from build123d import *

# Parameters (mm, degrees)
SKETCH1_R           = 17
BOSS_EXTRUDE1_DEPTH = 10


with BuildPart() as part:
    # Sketch1 → Boss-Extrude1 (new body)
    with BuildSketch(Plane(origin=(0, 0, 0), x_dir=(1, 0, 0), z_dir=(0, 1, 0))):
        with BuildLine():
            Line((-24.933996638, 20), (12.2, 20))
            ThreePointArc((12.2, 20), (-11.288251879, 45.878391012), (-39.314701644, 25))
            Line((-39.314701644, 25), (-164.9, 25))
            ThreePointArc((-164.9, 25), (-189.9, 0), (-164.9, -25))
            Line((-164.9, -25), (-39.314701644, -25))
            ThreePointArc((-39.314701644, -25), (-11.288251879, -45.878391012), (12.2, -20))
            Line((12.2, -20), (-24.933996638, -20))
            ThreePointArc((-24.933996638, -20), (-31.954004645, 0), (-24.933996638, 20))
        make_face()
        with Locations(Location((-164.9, 0, 0), (0, 0, 270))):
            Circle(SKETCH1_R, mode=Mode.SUBTRACT)
    extrude(amount=BOSS_EXTRUDE1_DEPTH)


solid = part.part
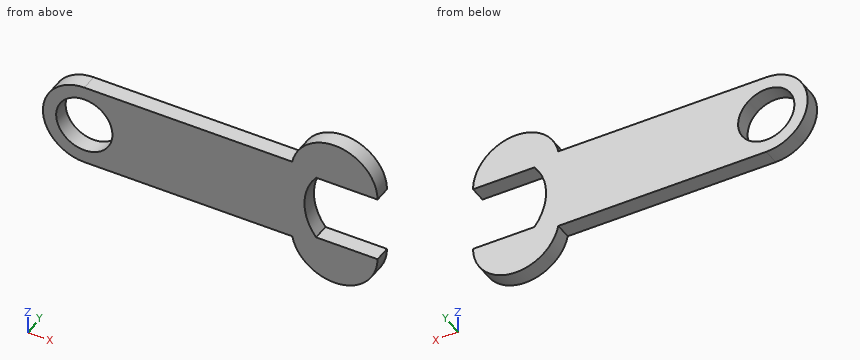
Design review of the part built by this model. Coordinates are the model's own, in mm. Give positions to 0.01 mm unless a question says otherwise; leave off trailing zeros. Loops run counter-clockwise (first coordinate to the right, second up) from the corner with the lowest first, then second, coordinate; pieces in that order, holes last. Notation, with made-up numbers: M -14,-5 L 0,-5 A28 cw 0,21 Z; hole C 52.5,12.25 d2. An arc over 180 degrees is marked long. One line per question, with ' | ' between items. Start each with the question number.
1. To check wall thickness, follow L1, parallel to Z at x = -14, y = 8.25; L2, parallel to Z at x = -120, y = 2; L3, parallel to X at y = 7.25, z = -14. State the ranges of each line that lie inside material, in increasing order.
2. Insertion check: P1, Ø2, axis at x = -84, y = 3.5, coming from the -Z side; P2, Ø8, axis at x = -30, z = 7, coming from the +Y side; P3, Ø5, axis at y = 8.5, z = 28.5, coming from the -X side; P4, Ø1.5, axis at y = 6.5, z = -21, coming from the +X side. Each pin has a flat end and moves straight along its axis. Give the tip position at first contact, or say it passes through.
3. Add section A-A (z = 0). Write out the cut boundary in (x, y), plus the area to 3 significant figures.
4. Add section B-B (y = 2.75). Write out the cut boundary in (x, z), plus the area to 3 significant figures.
5. Add section D-D (z = -35). Write out the cut boundary in (x, y), plus the area to 3 significant figures.
6. Add section C-C (x = -36). Write out the cut boundary in (y, z).
Worked out:
1) L1: z = -46 to -20, 20 to 46 | L2: z = -25 to 25 | L3: x = -185.61 to -174.54, -155.26 to -28.73
2) P1: stops at z = -25 | P2: stops at y = 10 | P3: stops at x = -39.1 | P4: stops at x = 12.2
3) outline: M -189.9,0 L -181.9,0 L -181.9,10 L -189.9,10 Z; M -147.9,0 L -31.95,0 L -31.95,10 L -147.9,10 Z | area: 1,240 mm²
4) outline: M -164.9,-25 L -39.31,-25 A26 ccw 12.2,-20 L -24.93,-20 A32 cw -24.93,20 L 12.2,20 A26 ccw -39.31,25 L -164.9,25 A25 ccw Z; hole C -164.9,0 d34 | area: 8,860 mm²
5) outline: M -35.04,0 L 7.44,0 L 7.44,10 L -35.04,10 Z | area: 425 mm²
6) outline: M 0,-33.53 L 10,-33.53 L 10,33.53 L 0,33.53 Z
